Geometry check sheet. Reference: the model listing, model coordinates, mm. Face numbers are marked on the shaded views. A direction names the side the tool comes from. Round coordinates to 2 decimals unless told otherwise and drop trailing zeros. Order: outer loops, then holes, each group sorted by start corner. A loop starts at its lowest first (then second) coordinate and runs counter-clockwise, first axis right, second up.
(1) Cross-section at B-B on x = 32.5. Enter the section's corners in (y, z).
(2) Cross-section at C-C on y = 21.5. Enter the section's corners in (x, z), and give its area (3 significant figures).
(3) Thickness scan on L1, parallel to Y at x = 7, z = 0 (3 decimals); L2, parallel to Y at x = 87, z = 0; L3, parallel to Z at x = 15.5, y = 0.5. Record the ranges inside material, lowest first.
(4) Draft check along Z on the marked faces 4 and 5. Enter one of: pulls with the +Z half, pulls with the -Z half, needs draft (parallel to the pull), parting line crosses it, or undercut.
(5) Cross-section at A-A on x = 16.5. Enter the section's corners in (y, z), and give its area (3 significant figures).
(6) Gauge pin test, flat ends, axial feed: P1, Ø12, axis at x = 12, z = 8, coming from the -Y side; P2, Ø7, axis at y = 0, z = 0, coming from the +X side; P3, Ø8, axis at x = 82, y = -3.5, coming from the +Z side. Record the tip position at first contact, or that the pin passes through.
(7) Set-up check for the marked faces 1, 2 and 3: record each of +Z, -Z, +X, -X, +Y, -Y from which the full face is reachable in a straight line by a thin tool's end or side.
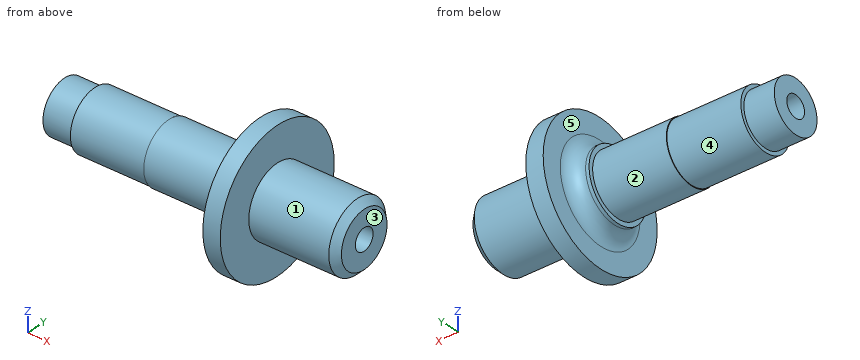
from build123d import *

# Parameters (mm, degrees)
SKETCH5_R          = 3.96875
CUT_EXTRUDE1_DEPTH = 28.575
SKETCH6_R          = 3.96875
CUT_EXTRUDE2_DEPTH = 33.782
CHAMFER1_SIZE      = 2.54


with BuildPart() as part:
    # Sketch4 → Revolve2 (revolve)
    with BuildSketch(Plane.XY):
        with BuildLine():
            Line((0, 0), (0, 9.525))
            Line((0, 9.525), (11.1125, 9.525))
            Line((11.1125, 9.525), (11.1125, 10.8712))
            Line((11.1125, 10.8712), (38.1, 10.8712))
            Line((38.1, 10.8712), (38.1, 11.1125))
            Line((38.1, 11.1125), (65.024, 11.1125))
            Line((65.024, 11.1125), (65.024, 12.7))
            Line((65.024, 12.7), (66.294, 12.7))
            ThreePointArc((66.294, 12.7), (69.886102448, 14.187897552), (71.374, 17.78))
            Line((71.374, 17.78), (71.374, 25.4))
            Line((71.374, 25.4), (77.724, 25.4))
            Line((77.724, 25.4), (77.724, 12.7))
            Line((77.724, 12.7), (109.474, 12.7))
            Line((109.474, 12.7), (109.474, 0))
            Line((109.474, 0), (0, 0))
        make_face()
    revolve(axis=Axis((109.474, 0, 0), (-1, 0, 0)))

    # Sketch5 → Cut-Extrude1 (cut)
    with BuildSketch(Plane.ZY):
        Circle(SKETCH5_R)
    extrude(amount=-CUT_EXTRUDE1_DEPTH, mode=Mode.SUBTRACT)

    # Sketch6 → Cut-Extrude2 (cut)
    with BuildSketch(Plane(origin=(109.474, 0, 0), x_dir=(0, 0, -1), z_dir=(1, 0, 0))):
        Circle(SKETCH6_R)
    extrude(amount=-CUT_EXTRUDE2_DEPTH, mode=Mode.SUBTRACT)

    # Chamfer1
    chamfer1_edges = [part.edges().sort_by_distance(p)[0] for p in [
        (109.474, -12.7, 0),
    ]]
    chamfer(chamfer1_edges, length=CHAMFER1_SIZE)


solid = part.part
Found:
1. outline: circle Ø21.74 at (0, 0)
2. outline: (71.37, -13.52) - (77.72, -13.52) - (77.72, 13.52) - (71.37, 13.52) - close
2. area: 172 mm2
3. L1: y = -9.525 to -3.969, 3.969 to 9.525
3. L2: y = -12.7 to -3.97, 3.97 to 12.7
3. L3: z = -10.86 to -3.94, 3.94 to 10.86
4. face 4: parting line crosses it
4. face 5: needs draft
5. outline: circle Ø21.74 at (0, 0); hole circle Ø7.94 at (0, 0)
5. area: 322 mm2
6. P1: stops at y = -10.69
6. P2: stops at x = 75.69
6. P3: stops at z = 12.7
7. face 1: +X
7. face 2: -X
7. face 3: +Z, -Z, +X, +Y, -Y
